Geometry check sheet. Reference: the model listing, model coordinates, mm. Coordinates: 2 decimals unless noted, no trailing zeros. Write each loop counter-clockwise with the first axis right and the second up, starting at its lowest first coordinate (ties: lowest second). Pieces come first, ordered by that corner, then holes.
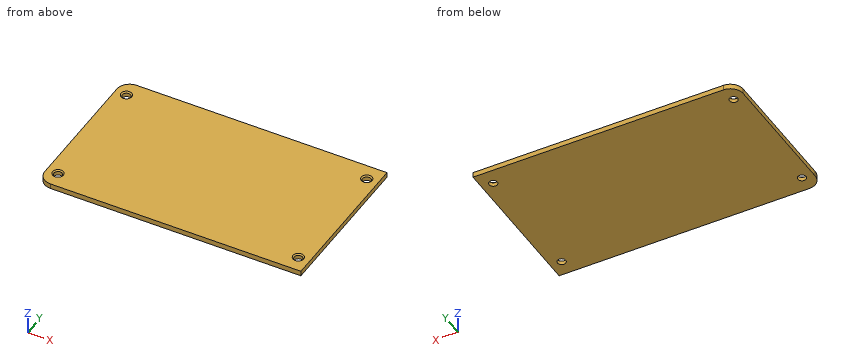
from build123d import *

# Parameters (mm, degrees)
F0_W     = 103.0236035585
F0_H     = 61.1
F0_R     = 1.6
F1_DEPTH = 2
F2_R     = 5
F3_SIZE  = 0.5


with BuildPart() as f1:
    # F0 (on Top) → F1 (new body)
    with BuildSketch(Plane.XY):
        Rectangle(F0_W, F0_H)
        with Locations((-47.05, -24.27)):
            Circle(F0_R, mode=Mode.SUBTRACT)
        with BuildLine():
            ThreePointArc((45.45, -24.27), (47.05, -22.67), (48.65, -24.27))
            ThreePointArc((48.65, -24.27), (47.05, -25.87), (45.45, -24.27))
        make_face(mode=Mode.SUBTRACT)
        with Locations((-47.05, 24.27)):
            Circle(F0_R, mode=Mode.SUBTRACT)
        with Locations((47.05, 24.27)):
            Circle(F0_R, mode=Mode.SUBTRACT)
    extrude(amount=F1_DEPTH)

    # F2
    f2_edges = [f1.edges().sort_by_distance(p)[0] for p in [
        (-51.511802, -30.55, 1),
        (-51.511802, 30.55, 1),
    ]]
    fillet(f2_edges, radius=F2_R)

    # F3
    f3_edges = [f1.edges().sort_by_distance(p)[0] for p in [
        (-48.65, -24.27, 2),
        (-48.65, 24.27, 2),
        (45.45, 24.27, 2),
        (48.65, -24.27, 2),
    ]]
    chamfer(f3_edges, length=F3_SIZE)


solid = f1.part
1. Gauge pin test, flat end, axial feed: pin 1 Ø2.5 at (x, y) = (47.05, -24.27) entering from -Z. Record the tip position at first contact, or that the pin passes through.
Computed values:
pin 1: passes through
2. Thickness scan on line 1 along Y through (x, z) = (47.05, 1.1); line 2 along Y through (x, z) = (-47.05, 0.4); line 3 along X through (y, z) = (-25, 1.75). Record the ranges inside material, lowest first.
Computed values:
line 1: y = -30.55 to -25.87, -22.67 to 22.67, 25.87 to 30.55
line 2: y = -30.52 to -25.87, -22.67 to 22.67, 25.87 to 30.52
line 3: x = -51.51 to -48.75, -45.35 to 45.35, 48.75 to 51.51
3. Sectioned sample at A-A, the plane x = 47.05. Record the boundary of the cut face in (y, z).
Computed values:
outline: (-30.55, 0) - (-25.87, 0) - (-25.87, 1.5) - (-26.37, 2) - (-30.55, 2) - close; (-22.67, 0) - (22.67, 0) - (22.67, 1.5) - (22.17, 2) - (-22.17, 2) - (-22.67, 1.5) - close; (25.87, 0) - (30.55, 0) - (30.55, 2) - (26.37, 2) - (25.87, 1.5) - close
4. Sectioned sample at B-B, the plane y = -24.27. Record the boundary of the cut face in (x, z).
Computed values:
outline: (-51.51, 0) - (-48.65, 0) - (-48.65, 1.5) - (-49.15, 2) - (-51.51, 2) - close; (-45.45, 0) - (45.45, 0) - (45.45, 1.5) - (44.95, 2) - (-44.95, 2) - (-45.45, 1.5) - close; (48.65, 0) - (51.51, 0) - (51.51, 2) - (49.15, 2) - (48.65, 1.5) - close
